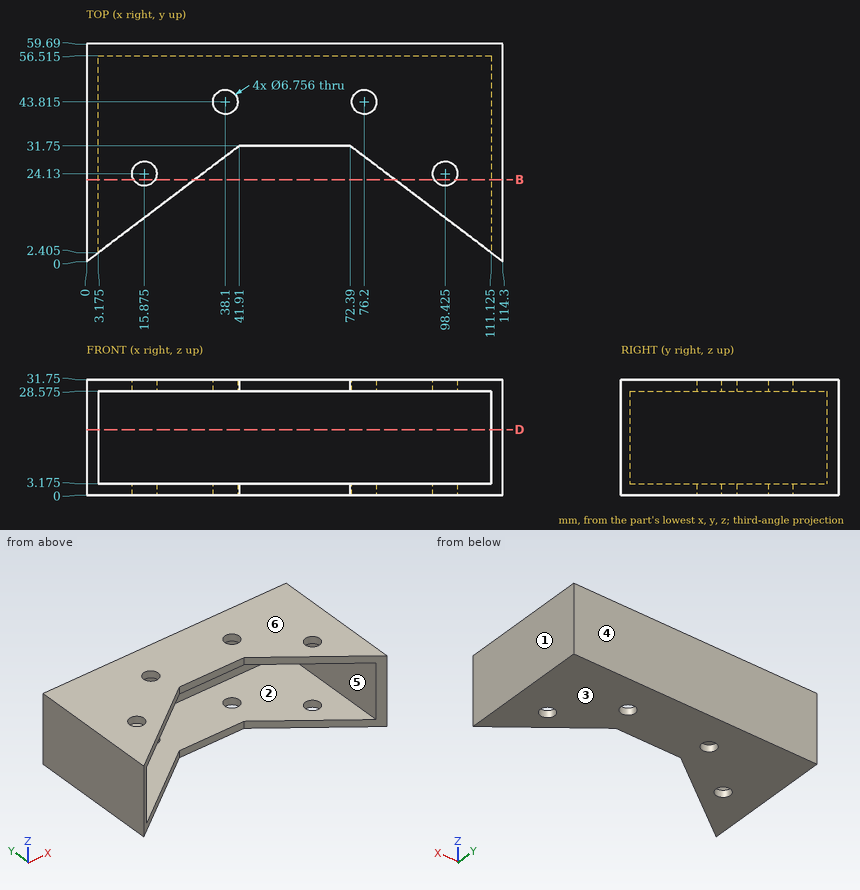
Answer from the drawing. Dimensions are ordinates in mm from the lowest x, y and z of the part. A direction names the side the tool comes from. Coordinates: 2 decimals unless noted, no trailing zeros. Order: outer loops, then holes, each group sorted by start corner. A loop starts at its lowest first (then second) coordinate and runs counter-clockwise, first axis right, second up. Notation, with made-up numbers: M -4.75,-17 L 17.25,-17 A28 cw 17.25,2 Z; hole C 33,-20 d7. An arc over 180 degrees is marked long. Put each result on its own line as item: value. Start each with the question number.
Item 1: The mould has two halves that part along Z. Classify the marked faces 3, 4, 5 and 6: +Z half, -Z half, draft (parallel to the pull), parting line (faces both ways), or undercut.
Item 2: Section D-D, the plane z = 18 is taken. Determine the outline of the cut face in (x, y) (1 decimal).
Item 3: Given pin 1 Ø6 at (x, y) = (15.875, 24.13) entering from +Z; pin 2 Ø1 at (x, z) = (63.5, 2) entering from -Y; pin 3 Ø8 at (x, z) = (25, 20) entering from -Y (3 decimals), each flat-ended and moving along its own axis, determine where each tip first touches the part or whether it passes through.
Item 4: Section B-B, the plane y = 22.5 is taken. Count the separate pieces of the cut face and the enclosed holes in it.
Item 5: Consider probe 1 along X at (y, z) = (10, 8) (1 decimal); probe 2 along Y at (x, z) = (102.5, 26.5) (1 decimal); probe 3 along X at (y, z) = (9.5, 29). Determine where each line is inside the solid, lowest interval first. Write a range as [from, to].
Item 6: For the marked faces 1 and 2, determine the directions among +Z, -Z, +X, -X, +Y, -Y from which every point of the face is accessible in a straight line to the end or side of a thin tool.
Computed:
1. face 3: -Z half
1. face 4: draft
1. face 5: undercut
1. face 6: +Z half
2. outline: M 0,0 L 3.2,2.4 L 3.2,56.5 L 111.1,56.5 L 111.1,2.4 L 114.3,0 L 114.3,59.7 L 0,59.7 Z
3. pin 1: passes through
3. pin 2: stops at y = 31.75
3. pin 3: stops at y = 56.515
4. separate pieces: 6
4. enclosed holes: 0
5. probe 1: x = [0, 3.2], [111.1, 114.3]
5. probe 2: y = [56.5, 59.7]
5. probe 3: x = [0, 12.54], [101.76, 114.3]
6. face 1: +Z, -Z, +X, +Y, -Y
6. face 2: -Y
